from build123d import *

# Parameters (mm, degrees)
BOSS_EXTRUDE1_DEPTH = 27.5
SKETCH2_R           = 1.75
BOSS_EXTRUDE2_DEPTH = 2


with BuildPart() as part:
    # Sketch1 → Boss-Extrude1 (new, symmetric)
    with BuildSketch(Plane.XY):
        Polygon((0, 0), (24, 0), (24, 11.191383796), align=None)
    extrude(amount=BOSS_EXTRUDE1_DEPTH, both=True)

    # Sketch2 → Boss-Extrude2 (add)
    with BuildSketch(Plane.XY.offset(27.5)):
        Polygon((24, 0), (24, 25), (14, 25), (0, 0), align=None)
        with Locations((19, 21)):
            Circle(SKETCH2_R, mode=Mode.SUBTRACT)
        with Locations((19, 15)):
            Circle(SKETCH2_R, mode=Mode.SUBTRACT)
    boss_extrude2 = extrude(amount=BOSS_EXTRUDE2_DEPTH)

    # Mirror1: Boss-Extrude2 across plane
    add(boss_extrude2.mirror(Plane.XY))


solid = part.part
Geometry: final body of the model. Coordinates: model frame, mm. A direction names the side the tool comes from. Coordinates: 2 decimals unless noted, no trailing zeros. Order: outer loops, then holes, each group sorted by start corner. A loop starts at its lowest first (then second) coordinate and runs counter-clockwise, first axis right, second up. Notation, with made-up numbers: M 82,24.25 L 104,24.25 A18 ccw 104,29.25 Z; hole C 47.25,76 d8. An arc over 180 degrees is marked long. One line per question, with ' | ' between items. Start each with the question number.
Item 1: Cut plane D-D, the plane x = 11.5. Return the cut outline in (y, z), then the cut area to 3 significant figures.
Item 2: Cut plane A-A, the plane y = 18. Return the cut outline in (x, z).
Item 3: Pin query (flat end, axial travel): pin 1 Ø5 at (x, z) = (11, -4.5) entering from +Y; pin 2 Ø4 at (y, z) = (11.5, -7.5) entering from -X. Return the tip coordinate at first contact, or that it passes through.
Item 4: Cut plane B-B, the plane y = 15. Return the cut outline in (x, z), then the cut area to 3 significant figures.
Item 5: Cut plane C-C, the plane x = 19. Return the cut outline in (y, z).
Item 6: Ray query, probe 1 along Y at (x, z) = (19, 29); probe 2 along Z at (x, y) = (6.25, 9.5); probe 3 along Y at (x, z) = (3.75, 3). Return the intervals inside material, ascending. Write a range as [from, to].
Item 7: Set-up query: faces 1 (the flat face through (12.168, 5.674, 0.385)), 2 (the flat face through (19, 25, 28)). Return all of +Z, -Z, +X, -X, +Y, -Y with unobstructed straight access to the full face (end or side cutting, diameter ignored); none if empty.
Item 8: Draft query along X for faces 3 (the flat face through (14, 13, -27.5)), 4 (the cylindrical face through (18.772, 22.735, 28.486)), 5 (the flat face through (7.098, 12.675, 28.486)). Return one class per face: released by +X, released by -X, zero draft, split by the parting line, or undercut.
A:
1) outline: M 0,-29.5 L 20.54,-29.5 L 20.54,-27.5 L 5.36,-27.5 L 5.36,27.5 L 20.54,27.5 L 20.54,29.5 L 0,29.5 Z | area: 377 mm2
2) outline: M 10.08,-29.5 L 24,-29.5 L 24,-27.5 L 10.08,-27.5 Z; M 10.08,27.5 L 24,27.5 L 24,29.5 L 10.08,29.5 Z
3) pin 1: stops at y = 6.3 | pin 2: stops at x = 20.37
4) outline: M 8.4,-29.5 L 17.25,-29.5 L 17.25,-27.5 L 8.4,-27.5 Z; M 8.4,27.5 L 17.25,27.5 L 17.25,29.5 L 8.4,29.5 Z; M 20.75,-29.5 L 24,-29.5 L 24,-27.5 L 20.75,-27.5 Z; M 20.75,27.5 L 24,27.5 L 24,29.5 L 20.75,29.5 Z | area: 48.4 mm2
5) outline: M 0,-29.5 L 13.25,-29.5 L 13.25,-27.5 L 8.86,-27.5 L 8.86,27.5 L 13.25,27.5 L 13.25,29.5 L 0,29.5 Z; M 16.75,-29.5 L 19.25,-29.5 L 19.25,-27.5 L 16.75,-27.5 Z; M 16.75,27.5 L 19.25,27.5 L 19.25,29.5 L 16.75,29.5 Z; M 22.75,-29.5 L 25,-29.5 L 25,-27.5 L 22.75,-27.5 Z; M 22.75,27.5 L 25,27.5 L 25,29.5 L 22.75,29.5 Z
6) probe 1: y = [0, 13.25], [16.75, 19.25], [22.75, 25] | probe 2: z = [-29.5, -27.5], [27.5, 29.5] | probe 3: y = [0, 1.75]
7) face 1: -X, +Y | face 2: +Z, -Z, +X, -X, +Y
8) face 3: zero draft | face 4: undercut | face 5: released by -X
